```python
from build123d import *

# Parameters (mm, degrees)
BOSS_EXTRUDE1_DEPTH = 3.175
BOSS_EXTRUDE2_DEPTH = 3.175


with BuildPart() as part:
    # Sketch1 → Boss-Extrude1 (new body)
    with BuildSketch(Plane.XY):
        Polygon((-13.5, 38.85), (-21.15, 38.85), (-21.15, -21.15), (-13.5, -21.15), (-13.5, -24.325), (-9.5, -24.325), (-9.5, -21.15), (-2, -21.15), (-2, -24.325), (2, -24.325), (2, -21.15), (9.5, -21.15), (9.5, -24.325), (13.5, -24.325), (13.5, -21.15), (21.15, -21.15), (21.15, 38.85), (13.5, 38.85), (13.5, 42.025), (9.5, 42.025), (9.5, 38.85), (2, 38.85), (2, 42.025), (-2, 42.025), (-2, 38.85), (-9.5, 38.85), (-9.5, 42.025), (-13.5, 42.025), align=None)
        with BuildLine():
            Line((-2.5, -15), (-2.5, 15))
            ThreePointArc((-2.5, 15), (0, 17.5), (2.5, 15))
            Line((2.5, 15), (2.5, -15))
            ThreePointArc((2.5, -15), (0, -17.5), (-2.5, -15))
        make_face(mode=Mode.SUBTRACT)
    extrude(amount=BOSS_EXTRUDE1_DEPTH)

    # Sketch2 → Boss-Extrude2 (add)
    with BuildSketch(Plane.XY.offset(3.175)):
        Polygon((21.19064, -21.19064), (21.19064, 38.89064), (13.54064, 38.89064), (13.54064, 42.06564), (9.45936, 42.06564), (9.45936, 38.89064), (2.04064, 38.89064), (2.04064, 42.06564), (-2.04064, 42.06564), (-2.04064, 38.89064), (-9.45936, 38.89064), (-9.45936, 42.06564), (-13.54064, 42.06564), (-13.54064, 38.89064), (-21.19064, 38.89064), (-21.19064, -21.19064), (-13.54064, -21.19064), (-13.54064, -24.36564), (-9.45936, -24.36564), (-9.45936, -21.19064), (-2.04064, -21.19064), (-2.04064, -24.36564), (2.04064, -24.36564), (2.04064, -21.19064), (9.45936, -21.19064), (9.45936, -24.36564), (13.54064, -24.36564), (13.54064, -21.19064), align=None)
        with BuildLine():
            Line((-2.45936, 15), (-2.45936, -15))
            ThreePointArc((-2.45936, -15), (0, -17.45936), (2.45936, -15))
            Line((2.45936, -15), (2.45936, 15))
            ThreePointArc((2.45936, 15), (0, 17.45936), (-2.45936, 15))
        make_face(mode=Mode.SUBTRACT)
    extrude(amount=-BOSS_EXTRUDE2_DEPTH)


solid = part.part
```
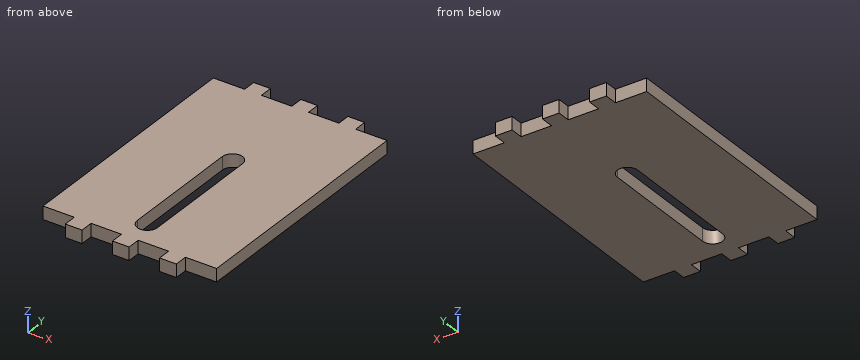
Verification items for the finished model (mm, model axes). Give positions to 0.01 mm unless a question says otherwise; leave off trailing zeros. Write each loop counter-clockwise with the first axis right and the second up, starting at its lowest first coordinate (ties: lowest second). Pieces come first, ordered by that corner, then holes. Notation, with made-up numbers: (34.25, -27.75) - (92.25, -27.75) arc R6 cw to (92.25, -18.75) - close; hole circle Ø2 at (-31, -20). An arc over 180 degrees is marked (long way). Put each result on its own line as item: value.
Q1. Depth check by flat-ended pin: P1, Ø1.6, axis at x = -17, z = 1, coming from the +Y side; P2, Ø1.6, axis at x = 7, z = 2, coming from the -Y side; P3, Ø1, axis at y = -23, z = 1.5, coming from the -X side. Enter the tip coordinate at first touch or a pass-through.
Result:
P1: y = 38.89
P2: y = -21.19
P3: x = -13.54
Q2. Scan lines: probe 1 along X at (y, z) = (39, 2.4); probe 2 along X at (y, z) = (-4, 1.6); probe 3 along Y at (x, z) = (15, 1.75). Record each from-to range of solid material in increasing order. Write a range as from..to.
Result:
probe 1: -13.54..-9.46, -2.04..2.04, 9.46..13.54
probe 2: -21.19..-2.46, 2.46..21.19
probe 3: -21.19..38.89
Q3. Section check B-B on y = -5. Record the cut outline in (x, z) (3 decimals), and give its area (3 significant figures).
Result:
outline: (-21.191, 0) - (-2.459, 0) - (-2.459, 3.175) - (-21.191, 3.175) - close; (2.459, 0) - (21.191, 0) - (21.191, 3.175) - (2.459, 3.175) - close
area: 119 mm2
Q4. Section check A-A on x = 0. Record the cut outline in (y, z) (3 decimals).
Result:
outline: (-24.366, 0) - (-17.459, 0) - (-17.459, 3.175) - (-24.366, 3.175) - close; (17.459, 0) - (42.066, 0) - (42.066, 3.175) - (17.459, 3.175) - close
